For this review, take the finished solid that the model builds, in its own axes (mm). Face numbers are marked on the shaded views. A direction names the side the tool comes from. Coordinates: 2 decimals unless noted, no trailing zeros. Loops run counter-clockwise (first coordinate to the right, second up) from the corner with the lowest first, then second, coordinate; pieces in that order, holes last. Notation, with made-up numbers: (-39, -22.5) -> (3, -22.5) arc R19 cw to (3, -12.5) -> close; hole circle Ø8 at (-38, 86). An arc over 180 degrees is marked (long way). Answer in a Markdown table with one row per item.
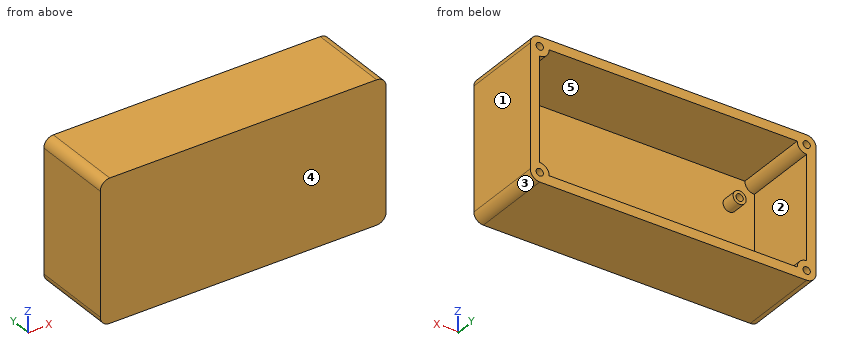
from build123d import *

# Parameters (mm, degrees)
SKETCH1_W           = 126.755144
SKETCH1_H           = 63.5
BOSS_EXTRUDE1_DEPTH = 2.54
SKETCH2_R           = 1.5875
BOSS_EXTRUDE2_DEPTH = 33
SKETCH2_4_W         = 126.755144
SKETCH2_4_H         = 63.5
CUT_EXTRUDE1_DEPTH  = 79.190658858
SKETCH4_R           = 2.8575
SKETCH4_R_2         = 1.5875
BOSS_EXTRUDE3_DEPTH = 6.35


with BuildPart() as part:
    # Sketch1 → Boss-Extrude1 (new body)
    with BuildSketch(Plane(origin=(0, 0, 0), x_dir=(1, 0, 0), z_dir=(0, 1, 0))):
        Rectangle(SKETCH1_W, SKETCH1_H)
    extrude(amount=BOSS_EXTRUDE1_DEPTH)

    # Sketch2 → Boss-Extrude2 (add)
    with BuildSketch(Plane(origin=(0, 2.54, 0), x_dir=(1, 0, 0), z_dir=(0, 1, 0))):
        with BuildLine():
            Line((-58.297572, -30.7975), (58.297572, -30.7975))
            ThreePointArc((58.297572, -30.7975), (61.216155239, -29.588583239), (62.425072, -26.67))
            Line((62.425072, -26.67), (62.425072, 26.67))
            ThreePointArc((62.425072, 26.67), (61.216155239, 29.588583239), (58.297572, 30.7975))
            Line((58.297572, 30.7975), (-58.297572, 30.7975))
            ThreePointArc((-58.297572, 30.7975), (-61.216155239, 29.588583239), (-62.425072, 26.67))
            Line((-62.425072, 26.67), (-62.425072, -26.67))
            ThreePointArc((-62.425072, -26.67), (-61.216155239, -29.588583239), (-58.297572, -30.7975))
        make_face()
        with Locations(Location((58.297572, 26.67, 0), (0, 0, 270))):
            Circle(SKETCH2_R, mode=Mode.SUBTRACT)
        with BuildLine():
            Line((58.297572, 22.5425), (58.297572, -22.5425))
            ThreePointArc((58.297572, -22.5425), (55.378988761, -23.751416761), (54.170072, -26.67))
            Line((54.170072, -26.67), (-54.170072, -26.67))
            ThreePointArc((-54.170072, -26.67), (-55.378988761, -23.751416761), (-58.297572, -22.5425))
            Line((-58.297572, -22.5425), (-58.297572, 22.5425))
            ThreePointArc((-58.297572, 22.5425), (-55.378988761, 23.751416761), (-54.170072, 26.67))
            Line((-54.170072, 26.67), (54.170072, 26.67))
            ThreePointArc((54.170072, 26.67), (55.378988761, 23.751416761), (58.297572, 22.5425))
        make_face(mode=Mode.SUBTRACT)
        with Locations(Location((-58.297572, -26.67, 0), (0, 0, 270))):
            Circle(SKETCH2_R, mode=Mode.SUBTRACT)
        with Locations(Location((58.297572, -26.67, 0), (0, 0, 270))):
            Circle(SKETCH2_R, mode=Mode.SUBTRACT)
        with Locations(Location((-58.297572, 26.67, 0), (0, 0, 270))):
            Circle(SKETCH2_R, mode=Mode.SUBTRACT)
    extrude(amount=BOSS_EXTRUDE2_DEPTH)

    # Sketch2_4 → Cut-Extrude1 (cut, through all)
    with BuildSketch(Plane(origin=(0, 2.54, 0), x_dir=(1, 0, 0), z_dir=(0, 1, 0))):
        Rectangle(SKETCH2_4_W, SKETCH2_4_H)
        with BuildLine():
            ThreePointArc((58.297572, 30.7975), (61.216155239, 29.588583239), (62.425072, 26.67))
            Line((62.425072, 26.67), (62.425072, -26.67))
            ThreePointArc((62.425072, -26.67), (61.216155239, -29.588583239), (58.297572, -30.7975))
            Line((58.297572, -30.7975), (-58.297572, -30.7975))
            ThreePointArc((-58.297572, -30.7975), (-61.216155239, -29.588583239), (-62.425072, -26.67))
            Line((-62.425072, -26.67), (-62.425072, 26.67))
            ThreePointArc((-62.425072, 26.67), (-61.216155239, 29.588583239), (-58.297572, 30.7975))
            Line((-58.297572, 30.7975), (58.297572, 30.7975))
        make_face(mode=Mode.SUBTRACT)
    extrude(amount=-CUT_EXTRUDE1_DEPTH, mode=Mode.SUBTRACT)

    # Sketch4 → Boss-Extrude3 (add)
    # profile 1 of 4: a face of its own
    with BuildSketch(Plane(origin=(0, 2.54, 0), x_dir=(1, 0, 0), z_dir=(0, 1, 0))):
        with Locations(Location((-47.498, 14.0589, 0), (0, 0, 270))):
            Circle(SKETCH4_R)
        with Locations(Location((-47.498, 14.0589, 0), (0, 0, 270))):
            Circle(SKETCH4_R_2, mode=Mode.SUBTRACT)
    # profile 2 of 4: a face of its own
    with BuildSketch(Plane(origin=(0, 2.54, 0), x_dir=(1, 0, 0), z_dir=(0, 1, 0))):
        with Locations(Location((-47.498, -14.0589, 0), (0, 0, 270))):
            Circle(SKETCH4_R)
        with Locations(Location((-47.498, -14.0589, 0), (0, 0, 270))):
            Circle(SKETCH4_R_2, mode=Mode.SUBTRACT)
    # profile 3 of 4: a face of its own
    with BuildSketch(Plane(origin=(0, 2.54, 0), x_dir=(1, 0, 0), z_dir=(0, 1, 0))):
        with Locations(Location((47.498, -14.0589, 0), (0, 0, 270))):
            Circle(SKETCH4_R)
        with Locations(Location((47.498, -14.0589, 0), (0, 0, 270))):
            Circle(SKETCH4_R_2, mode=Mode.SUBTRACT)
    # profile 4 of 4: a face of its own
    with BuildSketch(Plane(origin=(0, 2.54, 0), x_dir=(1, 0, 0), z_dir=(0, 1, 0))):
        with Locations(Location((47.498, 14.0589, 0), (0, 0, 270))):
            Circle(SKETCH4_R)
        with Locations(Location((47.498, 14.0589, 0), (0, 0, 270))):
            Circle(SKETCH4_R_2, mode=Mode.SUBTRACT)
    extrude(amount=BOSS_EXTRUDE3_DEPTH)


solid = part.part
Item 1: For the marked faces 1 and 2, list the 3-axis set-ups (+Z, -Z, +X, -X, +Y, -Y) from which the entire face can be reached by the end or side of a thin tool; tool diameter is ignored.
Worked answers:
| item | result |
|---|---|
| face 1 | +Z, -Z, +X, +Y, -Y |
| face 2 | +Y |
Item 2: Take a section at A-A, the plane x = -31. State the section outline as (y, z) points.
Worked answers:
| item | result |
|---|---|
| outline | (0, -30.8) -> (35.54, -30.8) -> (35.54, -26.67) -> (2.54, -26.67) -> (2.54, 26.67) -> (35.54, 26.67) -> (35.54, 30.8) -> (0, 30.8) -> close |
Item 3: Take a section at C-C, the plane y = 30. State the section outline as (x, z) points (1 decimal), and give its area (3 significant figures).
Worked answers:
| item | result |
|---|---|
| outline | (-62.4, -26.7) arc R4.1 ccw to (-58.3, -30.8) -> (58.3, -30.8) arc R4.1 ccw to (62.4, -26.7) -> (62.4, 26.7) arc R4.1 ccw to (58.3, 30.8) -> (-58.3, 30.8) arc R4.1 ccw to (-62.4, 26.7) -> close; hole circle Ø3.2 at (-58.3, -26.7); hole circle Ø3.2 at (-58.3, 26.7); hole (-58.3, -22.5) arc R4.1 cw to (-54.2, -26.7) -> (54.2, -26.7) arc R4.1 cw to (58.3, -22.5) -> (58.3, 22.5) arc R4.1 cw to (54.2, 26.7) -> (-54.2, 26.7) arc R4.1 cw to (-58.3, 22.5) -> close; hole circle Ø3.2 at (58.3, -26.7); hole circle Ø3.2 at (58.3, 26.7) |
| area | 1,480 mm² |
Item 4: Take a section at B-B, the plane z = -7.5. State the section outline as (x, y) points.
Worked answers:
| item | result |
|---|---|
| outline | (-62.43, 0) -> (62.43, 0) -> (62.43, 35.54) -> (58.3, 35.54) -> (58.3, 2.54) -> (-58.3, 2.54) -> (-58.3, 35.54) -> (-62.43, 35.54) -> close |
Item 5: Insertion check: pin 1 (1.9 mm diameter, centred on x = 47.5, z = 14.06, fed in from -Y); pin 2 (2.5 mm diameter, centred on x = 48, z = 15, fed in from +Y); pin 3 (1 mm diameter, centred on x = -48, z = -14.5, fed in from +Y). Each pin has a flat end and moves straight along its axis. Give the tip position at first contact, or say it passes through.
Worked answers:
| item | result |
|---|---|
| pin 1 | y = 0 |
| pin 2 | y = 8.89 |
| pin 3 | y = 2.54 |
Item 6: The part is to be moulded in two halves that separate along X. For the marked faces 3, 4 and 5, say which applies: +X half, -X half, draft (parallel to the pull), parting line (faces both ways), or undercut.
Worked answers:
| item | result |
|---|---|
| face 3 | +X half |
| face 4 | draft |
| face 5 | undercut |
Item 7: For L1, parallel to Z at x = 39.5, y = 18; L2, parallel to X at y = 24.5, z = 9; L3, parallel to Y at x = 47.5, z = 15, list the stretches that pass through material, from the lowest coordinate up.
Worked answers:
| item | result |
|---|---|
| L1 | -30.8 to -26.67, 26.67 to 30.8 |
| L2 | -62.43 to -58.3, 58.3 to 62.43 |
| L3 | 0 to 2.54 |
